Could you check a few things on this model? Use its own coordinates, in mm. A direction names the side the tool comes from. Round coordinates to 2 decimals unless told otherwise and drop trailing zeros. Loops run counter-clockwise (first coordinate to the right, second up) from the corner with the lowest first, then second, coordinate; pieces in that order, holes last. Notation, with made-up numbers: (8.25, 31.5) -> (24.25, 31.5) arc R15 cw to (24.25, 58.5) -> close; hole circle Ø2 at (-39.5, 72.5). An arc over 180 degrees is marked (long way). One line per item, written item: value.
```python
from build123d import *

# Parameters (mm, degrees)
F0_W           = 177.8
F0_H           = 76.2
F1_DEPTH       = 19.05
F3_DEPTH       = 25.4
F5_DEPTH       = 6.35
F7_D           = 8.636
F7_CBORE_D     = 12.7
F7_CBORE_DEPTH = 9.652


with BuildPart() as f1:
    # F0 (on Front) → F1 (new body)
    with BuildSketch(Plane.XZ):
        with Locations((88.9, 38.1)):
            Rectangle(F0_W, F0_H)
    extrude(amount=F1_DEPTH)

    # F2 (on face) → F3 (cut)
    with BuildSketch(Plane.XZ.offset(19.05)):
        with BuildLine():
            ThreePointArc((22.352, 34.925), (23.281936, 32.679936), (25.527, 31.75))
            Line((25.527, 31.75), (152.527, 31.75))
            ThreePointArc((152.527, 31.75), (154.772064, 32.679936), (155.702, 34.925))
            Line((155.702, 34.925), (155.702, 41.3004))
            ThreePointArc((155.702, 41.3004), (154.772064, 43.545464), (152.527, 44.4754))
            Line((152.527, 44.4754), (25.527, 44.4754))
            ThreePointArc((25.527, 44.4754), (23.281936, 43.545464), (22.352, 41.3004))
            Line((22.352, 41.3004), (22.352, 34.925))
        make_face()
    extrude(amount=-F3_DEPTH, mode=Mode.SUBTRACT)

    # F4 (on face) → F5 (cut)
    with BuildSketch(Plane.XZ.offset(19.05)):
        with BuildLine():
            Line((155.575, 47.6504), (22.225, 47.6504))
            ThreePointArc((22.225, 47.6504), (19.979936, 46.720464), (19.05, 44.4754))
            Line((19.05, 44.4754), (19.05, 31.75))
            ThreePointArc((19.05, 31.75), (19.979936, 29.504936), (22.225, 28.575))
            Line((22.225, 28.575), (155.575, 28.575))
            ThreePointArc((155.575, 28.575), (157.820064, 29.504936), (158.75, 31.75))
            Line((158.75, 31.75), (158.75, 44.4754))
            ThreePointArc((158.75, 44.4754), (157.820064, 46.720464), (155.575, 47.6504))
        make_face()
    extrude(amount=-F5_DEPTH, mode=Mode.SUBTRACT)

    # F7 (through all)
    with Locations(Plane.XZ.offset(19.05)):
        with Locations((9.525, 15.875), (9.525, 60.325), (168.275, 60.325), (168.275, 15.875)):
            CounterBoreHole(F7_D / 2, F7_CBORE_D / 2, F7_CBORE_DEPTH)


solid = f1.part
```
Item 1: If we mould it in two halves opening along X, with no side actions, what happens to faces 4 (the face through (88, -9, 0)), 5 (the face through (0, -9, 38)), 6 (the face through (7.533, -4.633, 12.044))? For each: released by +X, released by -X, zero draft, split by the parting line, or undercut.
Output:
face 4: zero draft
face 5: released by -X
face 6: undercut
Item 2: If we section it at A-A on x = 123: List the corners of the cut face in (y, z) for me (3 decimals), plus the area to 3 significant figures.
Output:
outline: (-19.05, 0) -> (0, 0) -> (0, 31.75) -> (-12.7, 31.75) -> (-12.7, 28.575) -> (-19.05, 28.575) -> close; (-19.05, 47.65) -> (-12.7, 47.65) -> (-12.7, 44.475) -> (0, 44.475) -> (0, 76.2) -> (-19.05, 76.2) -> close
area: 1,170 mm²
Item 3: I need wall thicknesses on line 1 (Z direction, x = 138.5, y = -8.75); line 2 (X direction, y = -11.25, z = 10); line 3 (Z direction, x = 12, y = -1.5). Which ranges of each line are inside material? Lowest first, please. Write a range as from..to.
Output:
line 1: z = 0..31.75, 44.48..76.2
line 2: x = 0..7.12, 11.93..165.87, 170.68..177.8
line 3: z = 0..12.34, 19.41..56.79, 63.86..76.2
Item 4: Will these pins go through, and if not, where does the flat tip stop? pin 1 Ø8 at (x, z) = (168.275, 60.325) entering from +Y; pin 2 Ø4 at (x, z) = (7, 17.5) entering from -Y.
Output:
pin 1: passes through
pin 2: stops at y = -9.4
Item 5: For faces 1 (the face through (23, -6, 33)), 2 (the face through (14, -9.398, 15)), 3 (the face through (88, 0, 47)), which set-ups out of +Z, -Z, +X, -X, +Y, -Y let a thin tool reach every point of the face, with its end or its side?
Output:
face 1: +Y, -Y
face 2: -Y
face 3: +Z, -Z, +X, -X, +Y
Item 6: If we section it at B-B on y = -14.5: List the corners of the cut face in (x, z) for me (3 decimals).
Output:
outline: (0, 0) -> (177.8, 0) -> (177.8, 76.2) -> (0, 76.2) -> close; hole circle Ø12.7 at (9.525, 15.875); hole circle Ø12.7 at (9.525, 60.325); hole (19.05, 31.75) arc R3.175 ccw to (22.225, 28.575) -> (155.575, 28.575) arc R3.175 ccw to (158.75, 31.75) -> (158.75, 44.475) arc R3.175 ccw to (155.575, 47.65) -> (22.225, 47.65) arc R3.175 ccw to (19.05, 44.475) -> close; hole circle Ø12.7 at (168.275, 15.875); hole circle Ø12.7 at (168.275, 60.325)
